from build123d import *

# Parameters (mm, degrees)
SKETCH1_R           = 2.54
BOSS_EXTRUDE1_DEPTH = 3.175
FILLET1_R           = 3.175


with BuildPart() as part:
    # Sketch1 → Boss-Extrude1 (new body)
    with BuildSketch(Plane.XY):
        Polygon((-12.7, -12.7), (12.7, -12.7), (12.7, 38.1), (-63.5, 100.883206633), (-63.5, 139.7), (-88.9, 139.7), (-88.9, 88.9), (-12.7, 26.116793367), align=None)
        with Locations((0, 25.4)):
            Circle(SKETCH1_R, mode=Mode.SUBTRACT)
        Circle(SKETCH1_R, mode=Mode.SUBTRACT)
        with Locations((-76.2, 127)):
            Circle(SKETCH1_R, mode=Mode.SUBTRACT)
        with Locations((-76.2, 101.6)):
            Circle(SKETCH1_R, mode=Mode.SUBTRACT)
    extrude(amount=BOSS_EXTRUDE1_DEPTH)

    # Fillet1
    fillet1_edges = [part.edges().sort_by_distance(p)[0] for p in [
        (-88.9, 88.9, 1.5875),
        (-88.9, 139.7, 1.5875),
        (-63.5, 139.7, 1.5875),
        (-63.5, 100.883206633, 1.5875),
        (12.7, 38.1, 1.5875),
        (12.7, -12.7, 1.5875),
        (-12.7, -12.7, 1.5875),
        (-12.7, 26.116793367, 1.5875),
    ]]
    fillet(fillet1_edges, radius=FILLET1_R)


solid = part.part
Check sheet for the modelled part. Datum: model origin and axes. Units: mm. A direction names the side the tool comes from. Give positions to 0.01 mm unless a question says otherwise; leave off trailing zeros. Loops run counter-clockwise (first coordinate to the right, second up) from the corner with the lowest first, then second, coordinate; pieces in that order, holes last. Notation, with made-up numbers: M 45,-18 L 82,-18 A24 cw 82,10 Z; hole C 13.5,62 d3. An arc over 180 degrees is marked long. Answer as a JSON object with one key per item and string values. Group by question number.
Q1. Cross-section at D-D on y = 115. Record the cut outline in (x, z) (3 decimals), then the cut area to 3 significant figures.
Q2. Cross-section at B-B on z = 1.65. Give the number of separate pieces and of enclosed holes in the cut face, then the cut area to 3 significant figures.
Q3. Release check for a two-part mould opening along Y. For faces 1 (the cylindrical face through (11.75, -11.79, 1.61)), 2 (the cylindrical face through (-78.216, 125.454, 1.565)), 3 (the cylindrical face through (-64.41, 138.75, 1.61)), 4 (the cylindrical face through (-76.75, 99.12, 1.57)) record: released by +Y, released by -Y, zero draft, split by the parting line, or undercut.
Q4. Access from +Z, -Z, +X, -X, +Y, -Y to the whole of each face (thin tool, end or side, straight path). Record for faces 5 (the flat face through (-12.7, 8, 2)), 6 (the flat face through (-63.5, 119, 2)), 7 (the cylindrical face through (-87.99, 138.75, 1.61)).
Q5. Cross-section at C-C on x = 0. Record the cut outline in (y, z) (3 decimals), then the cut area to 3 significant figures.
Q6. Material ranges on line 1 along Y through (x, z) = (-76.2, 2); line 2 along Y through (x, z) = (1, 0.2); line 3 along X through (y, z) = (111.5, 2.95), recorded low to high. Write a range as [from, to].
Q7. Go/stop test with flat-tipped pins: P1, Ø1, axis at y = 12, z = 1.5, coming from the -X side; P2, Ø1, axis at y = 90.5, z = 2, coming from the +X side. Record where each tip stops, or that it passes through.
Q8. Cross-section at A-A on y = 0. Record the cut outline in (x, z) (3 decimals), then the cut area to 3 significant figures.
Evaluation:
{
 "1": {"outline": "M -88.9,0 L -63.5,0 L -63.5,3.175 L -88.9,3.175 Z", "area": "80.6 mm2"},
 "2": {"separate pieces": "1", "enclosed holes": "4", "area": "4,690 mm2"},
 "3": {"face 1": "released by -Y", "face 2": "undercut", "face 3": "released by +Y", "face 4": "undercut"},
 "4": {"face 5": "+Z, -Z, -X, -Y", "face 6": "+Z, -Z, +X, +Y", "face 7": "+Z, -Z, -X, +Y"},
 "5": {"outline": "M -12.7,0 L -2.54,0 L -2.54,3.175 L -12.7,3.175 Z; M 2.54,0 L 22.86,0 L 22.86,3.175 L 2.54,3.175 Z; M 27.94,0 L 48.564,0 L 48.564,3.175 L 27.94,3.175 Z", "area": "162 mm2"},
 "6": {"line 1": "y = [78.44, 99.06], [104.14, 124.46], [129.54, 139.7]", "line 2": "y = [-12.7, -2.33], [2.33, 23.07], [27.73, 47.74]", "line 3": "x = [-88.9, -63.5]"},
 "7": {"P1": "stops at x = -12.7", "P2": "stops at x = -50.29"},
 "8": {"outline": "M -12.7,0 L -2.54,0 L -2.54,3.175 L -12.7,3.175 Z; M 2.54,0 L 12.7,0 L 12.7,3.175 L 2.54,3.175 Z", "area": "64.5 mm2"}
}
